Check sheet for the modelled part. Datum: model origin and axes. Units: mm. A direction names the side the tool comes from. Give positions to 0.01 mm unless a question says otherwise; leave off trailing zeros. Order: outer loops, then holes, each group sorted by start corner. A loop starts at its lowest first (then second) coordinate and runs counter-clockwise, first axis right, second up. Notation, with made-up numbers: (34, 34.25) - (86, 34.25) arc R25 cw to (86, 56.25) - close; hole circle Ø8 at (0, 31). An arc over 180 degrees is marked (long way). Answer in a Markdown table with one row per item.
from build123d import *

# Parameters (mm, degrees)
F0_W     = 20
F0_H     = 20
F0_R     = 8.15
F1_DEPTH = 6


with BuildPart() as f1:
    # F0 (on Front) → F1 (new body)
    with BuildSketch(Plane.XZ):
        Polygon((-10, 10), (10, 10), (20, 27.320508), (10, 44.641016), (-10, 44.641016), (-20, 27.320508), align=None)
        Polygon((4.99408, 35.970508), (9.98816, 27.320508), (4.99408, 18.670508), (-4.99408, 18.670508), (-9.98816, 27.320508), (-4.99408, 35.970508), align=None, mode=Mode.SUBTRACT)
        Rectangle(F0_W, F0_H)
        Circle(F0_R, mode=Mode.SUBTRACT)
        Polygon((20, -27.320508), (10, -10), (-10, -10), (-20, -27.320508), (-10, -44.641016), (10, -44.641016), align=None)
        Polygon((4.99408, -35.970508), (-4.99408, -35.970508), (-9.98816, -27.320508), (-4.99408, -18.670508), (4.99408, -18.670508), (9.98816, -27.320508), align=None, mode=Mode.SUBTRACT)
    extrude(amount=F1_DEPTH)


solid = f1.part
(1) Cross-section at A-A, the plane z = 0. Record the cut outline in (x, y), then the cut area to 3 significant figures.
Geometry says:
| item | result |
|---|---|
| outline | (-10, -6) - (-8.15, -6) - (-8.15, 0) - (-10, 0) - close; (8.15, -6) - (10, -6) - (10, 0) - (8.15, 0) - close |
| area | 22.2 mm² |
(2) Access from +Z, -Z, +X, -X, +Y, -Y to the whole of each face (thin tool, end or side, straight path). Record for faces 4 (the flat face through (-15.07, -2.96, -35.86)), 5 (the flat face through (-15.07, -2.96, 18.78)), 6 (the flat face through (7.53, -2.96, 23.06)).
Geometry says:
| item | result |
|---|---|
| face 4 | -Z, -X, +Y, -Y |
| face 5 | -X, +Y, -Y |
| face 6 | +Y, -Y |
(3) Cross-section at C-C, the plane x = 0. Record the cut outline in (y, z), then the cut area to 3 significant figures.
Geometry says:
| item | result |
|---|---|
| outline | (-6, -44.64) - (0, -44.64) - (0, -35.97) - (-6, -35.97) - close; (-6, -18.67) - (0, -18.67) - (0, -8.15) - (-6, -8.15) - close; (-6, 8.15) - (0, 8.15) - (0, 18.67) - (-6, 18.67) - close; (-6, 35.97) - (0, 35.97) - (0, 44.64) - (-6, 44.64) - close |
| area | 230 mm² |
(4) Gauge pin test, flat ends, axial feed: P1, Ø1, axis at y = -1, z = -35.5, coming from the +X side; P2, Ø1.8, axis at y = -3, z = -4.5, coming from the +X side; P3, Ø12, axis at x = 5, z = 20.5, coming from the +Y side; P4, Ø13, axis at x = 0, z = 0, coming from the +Y side. Record the tip position at first contact, or that the pin passes through.
Geometry says:
| item | result |
|---|---|
| P1 | x = 15.57 |
| P2 | x = 10 |
| P3 | y = 0 |
| P4 | through |
(5) Cross-section at D-D, the plane x = -12.5. Record the cut outline in (y, z), then the cut area to 3 significant figures.
Geometry says:
| item | result |
|---|---|
| outline | (-6, -40.31) - (0, -40.31) - (0, -14.33) - (-6, -14.33) - close; (-6, 14.33) - (0, 14.33) - (0, 40.31) - (-6, 40.31) - close |
| area | 312 mm² |
(6) Cross-section at B-B, the plane y = -1.65. Record the cut outline in (x, z).
Geometry says:
| item | result |
|---|---|
| outline | (-20, -27.32) - (-10, -44.64) - (10, -44.64) - (20, -27.32) - (10, -10) - (10, 10) - (20, 27.32) - (10, 44.64) - (-10, 44.64) - (-20, 27.32) - (-10, 10) - (-10, -10) - close; hole (-9.99, -27.32) - (-4.99, -35.97) - (4.99, -35.97) - (9.99, -27.32) - (4.99, -18.67) - (-4.99, -18.67) - close; hole (-9.99, 27.32) - (-4.99, 18.67) - (4.99, 18.67) - (9.99, 27.32) - (4.99, 35.97) - (-4.99, 35.97) - close; hole circle Ø16.3 at (0, 0) |
(7) Thickness scan on L1, parallel to Z at x = -0.5, y = -1.4; L2, parallel to X at y = -0.4, z = 0.5; L3, parallel to Z at x = 4, y = -4.7. Record the ranges inside material, lowest first.
Geometry says:
| item | result |
|---|---|
| L1 | -44.64 to -35.97, -18.67 to -8.13, 8.13 to 18.67, 35.97 to 44.64 |
| L2 | -10 to -8.13, 8.13 to 10 |
| L3 | -44.64 to -35.97, -18.67 to -7.1, 7.1 to 18.67, 35.97 to 44.64 |
(8) Mould release check, pull along Z, two halves, no side actions. Record for faces 1 (the flat face through (14.93, -2.96, -36.1)), 2 (the flat face through (-14.93, -2.96, 36.1)), 3 (the flat face through (14.93, -2.96, 18.54)): pulls with the +Z half, pulls with the -Z half, needs draft (parallel to the pull), parting line crosses it, or undercut.
Geometry says:
| item | result |
|---|---|
| face 1 | pulls with the -Z half |
| face 2 | pulls with the +Z half |
| face 3 | undercut |
